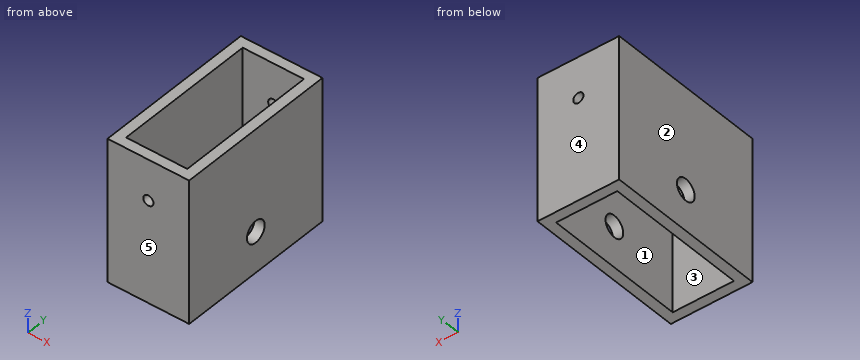
Autodesk Inventor part; units mm, degrees
ref_plane "YZ Plane" through (0, 0, 0) normal (1, 0, 0) x (0, 1, 0)
ref_plane "XZ Plane" through (0, 0, 0) normal (0, 1, 0) x (-1, 0, 0)
ref_plane "XY Plane" through (0, 0, 0) normal (0, 0, 1) x (1, 0, 0)
sketch "Sketch1" plane through (0, 0, 0) normal (0, 0, 1) x (1, 0, 0)
  line L0 (0, 0) -> (25.4, 0)
  line L1 (25.4, 0) -> (25.4, 50.8)
  line L2 (25.4, 50.8) -> (0, 50.8)
  line L3 (0, 50.8) -> (0, 0)
  dimension "d0" = 25.4
  dimension "d1" = 50.8
extrude "Extrusion1" add sketch "Sketch1" along normal blind 44.45
shell "Shell2" thickness 3.175 removed faces 2 at (8.4667, 16.9333, 0) at (8.4667, 16.9333, 44.45)
sketch "Sketch2" plane through (25.4, 0, 0) normal (1, 0, 0) x (0, 0, -1)
  circle A0 centre (-12.7, 25.4) radius 3.3782
  line L0 (0, 0) -> (0, 50.8)
  line L1 (0, 50.8) -> (-44.45, 50.8)
  dimension "d6" = 12.7
  dimension "d7" = 6.7564
  dimension "d8" = 25.4
extrude "Extrusion2" cut sketch "Sketch2" against normal blind 63.5
sketch "Sketch3" plane through (0, 50.8, 0) normal (0, 1, 0) x (1, 0, 0)
  line L0 (25.4, -44.45) -> (0, -44.45)
  line L1 (12.7, -44.45) -> (12.7, -31.75)
  circle A0 centre (12.7, -31.75) radius 1.5875
  point P0 (0, 0)
  dimension "d11" = 12.7
  dimension "d12" = 3.175
extrude "Extrusion3" cut sketch "Sketch3" against normal blind 63.5
properties part number "bumper beam" material "Aluminum 6061"
Design review of the part built by this model. Coordinates are the model's own, in mm. Face numbers are marked on the shaded views. A direction names the side the tool comes from. Round coordinates to 2 decimals unless told otherwise and drop trailing zeros. Write each loop counter-clockwise with the first axis right and the second up, starting at its lowest first coordinate (ties: lowest second). Pieces come first, ordered by that corner, then holes. Notation, with made-up numbers: (69, -34.75) -> (76, -34.75) arc R11 ccw to (76, -22.75) -> close; hole circle Ø10 at (11, -29.75). An arc over 180 degrees is marked (long way). Answer in a Markdown table with one row per item.
Q1. Take a section at A-A, the plane y = 45.5. State the section outline as (x, z) points (3 decimals), then the cut area to 3 significant figures.
The answers:
| item | result |
|---|---|
| outline | (0, 0) -> (3.175, 0) -> (3.175, 44.45) -> (0, 44.45) -> close; (22.225, 0) -> (25.4, 0) -> (25.4, 44.45) -> (22.225, 44.45) -> close |
| area | 282 mm² |
Q2. For the marked faces 1 and 2, list the 3-axis set-ups (+Z, -Z, +X, -X, +Y, -Y) from which the entire face can be reached by the end or side of a thin tool; tool diameter is ignored.
The answers:
| item | result |
|---|---|
| face 1 | +Z, -Z |
| face 2 | +Z, -Z, -X, +Y, -Y |
Q3. Take a section at B-B, the plane z = 31.75. State the section outline as (x, y) points (1 decimal), then the cut area to 3 significant figures.
The answers:
| item | result |
|---|---|
| outline | (0, 0) -> (11.1, 0) -> (11.1, 3.2) -> (3.2, 3.2) -> (3.2, 47.6) -> (11.1, 47.6) -> (11.1, 50.8) -> (0, 50.8) -> close; (14.3, 0) -> (25.4, 0) -> (25.4, 50.8) -> (14.3, 50.8) -> (14.3, 47.6) -> (22.2, 47.6) -> (22.2, 3.2) -> (14.3, 3.2) -> close |
| area | 423 mm² |
Q4. Take a section at D-D, the plane x = 7. State the section outline as (y, z) points (3 decimals).
The answers:
| item | result |
|---|---|
| outline | (0, 0) -> (3.175, 0) -> (3.175, 44.45) -> (0, 44.45) -> close; (47.625, 0) -> (50.8, 0) -> (50.8, 44.45) -> (47.625, 44.45) -> close |
Q5. To check wall thickness, follow L1, parallel to Y at x = 22, z = 33 (3 decimals); L2, parallel to X at y = 43, z = 8 (3 decimals); L3, parallel to X at y = 1.2, z = 31.75. State the ranges of each line that lie inside material, in increasing order. Write a range as [from, to].
The answers:
| item | result |
|---|---|
| L1 | [0, 3.175], [47.625, 50.8] |
| L2 | [0, 3.175], [22.225, 25.4] |
| L3 | [0, 11.11], [14.29, 25.4] |
Q6. Draft analysis for pull direction Y (two halves, no side actions). For the marked faces 3, 4 and 5, state which applies: +Y half, -Y half, draft (parallel to the pull), parting line (faces both ways), or undercut.
The answers:
| item | result |
|---|---|
| face 3 | undercut |
| face 4 | +Y half |
| face 5 | -Y half |
Q7. Take a section at C-C, the plane x = 12.7. Count the separate pieces of the cut face and the enclosed holes in it, then the cut area to 3 significant figures.
The answers:
| item | result |
|---|---|
| separate pieces | 4 |
| enclosed holes | 0 |
| area | 262 mm² |
